from build123d import *

# Parameters (mm, degrees)
BOX010_W                = 100
BOX010_H                = 100
BOX010_DEPTH            = 20
CYLINDER010_R           = 6
CYLINDER010_DEPTH       = 60
CYLINDER011_R           = 2.1
CYLINDER011_DEPTH       = 40
BOX009_W                = 40
BOX009_H                = 30
BOX009_DEPTH            = 5
FILLET002_R             = 10
CYLINDER013_R           = 1
CYLINDER013_DEPTH       = 60
CYLINDER014_R           = 1
CYLINDER014_DEPTH       = 40
BODY005_PLACEMENT_ANGLE = 90
CYLINDER015_R           = 1
CYLINDER015_DEPTH       = 60
CYLINDER016_R           = 1
CYLINDER016_DEPTH       = 40
BODY006_PLACEMENT_ANGLE = 90
BOX008_W                = 22
BOX008_H                = 22
BOX008_DEPTH            = 50
CUT003_PLACEMENT_ANGLE  = 15


with BuildPart() as base_cube002:
    # Box010 → Box010 (new body)
    with BuildSketch(Plane(origin=(-8, -50, -20), x_dir=(1, 0, 0), z_dir=(0, 0, 1))):
        with Locations((50, 50)):
            Rectangle(BOX010_W, BOX010_H)
    extrude(amount=BOX010_DEPTH)


with BuildPart() as cone005:
    # Cone005 → Cone005 (revolve)
    with BuildSketch(Plane.XZ):
        Polygon((0, 0), (2.1, 0), (6, 4), (0, 4), align=None)
    revolve(axis=Axis((0, 0, 0), (0, 0, 1)))


with BuildPart() as cylinder010:
    # Cylinder010 → Cylinder010 (new body)
    with BuildSketch(Plane.XY.offset(4)):
        Circle(CYLINDER010_R)
    extrude(amount=CYLINDER010_DEPTH)


with BuildPart() as extraction_fusion001:
    # Cylinder011 → Cylinder011 (new body)
    with BuildSketch(Plane.XY.offset(-40)):
        Circle(CYLINDER011_R)
    extrude(amount=CYLINDER011_DEPTH)

    # Fusion012: union Cone005, Cylinder010
    add(cone005.part)
    add(cylinder010.part)


with BuildPart() as extraction_fusion001_1:
    # Fusion012 placement: moved
    add(extraction_fusion001.part.moved(Location((0, 0, 5))))


with BuildPart() as extraction_fusion001_2:
    # Body008 placement: moved
    add(extraction_fusion001_1.part.moved(Location((-17, 0, -5))))

    # Fusion014: union base cube002
    add(base_cube002.part)


with BuildPart() as base_cube_fillet001:
    # Box009 → Box009 (new body)
    with BuildSketch(Plane(origin=(-25, -15, 0), x_dir=(1, 0, 0), z_dir=(0, 0, 1))):
        with Locations((20, 15)):
            Rectangle(BOX009_W, BOX009_H)
    extrude(amount=BOX009_DEPTH)

    # Fillet002
    fillet002_edges = [base_cube_fillet001.edges().sort_by_distance(p)[0] for p in [
        (-25, -15, 2.5),
        (-25, 15, 2.5),
        (15, -15, 2.5),
        (15, 15, 2.5),
    ]]
    fillet(fillet002_edges, radius=FILLET002_R)


with BuildPart() as screw_hole_cylinder001:
    # Cylinder013 → Cylinder013 (new body)
    with BuildSketch(Plane.XY):
        Circle(CYLINDER013_R)
    extrude(amount=CYLINDER013_DEPTH)


with BuildPart() as m3_screw_hole_fusion_clone002:
    # Cylinder014 → Cylinder014 (new body)
    with BuildSketch(Plane.XY.offset(-40)):
        Circle(CYLINDER014_R)
    extrude(amount=CYLINDER014_DEPTH)

    # Fusion011: union screw hole cylinder001
    add(screw_hole_cylinder001.part)


with BuildPart() as m3_screw_hole_fusion_clone002_1:
    # Fusion011 placement: moved
    add(m3_screw_hole_fusion_clone002.part.moved(Location((0, 0, 5))))


with BuildPart() as m3_screw_hole_fusion_clone002_2:
    # Body005 placement: moved
    add(m3_screw_hole_fusion_clone002_1.part.moved(Location((11, 26, 37))).rotate(Axis((11, 26, 37), (1, 0, 0)), BODY005_PLACEMENT_ANGLE))


with BuildPart() as cylinder015:
    # Cylinder015 → Cylinder015 (new body)
    with BuildSketch(Plane.XY):
        Circle(CYLINDER015_R)
    extrude(amount=CYLINDER015_DEPTH)


with BuildPart() as m3_hole_fusion001:
    # Cylinder016 → Cylinder016 (new body)
    with BuildSketch(Plane.XY.offset(-40)):
        Circle(CYLINDER016_R)
    extrude(amount=CYLINDER016_DEPTH)

    # Fusion016: union Cylinder015
    add(cylinder015.part)


with BuildPart() as m3_hole_fusion001_1:
    # Fusion016 placement: moved
    add(m3_hole_fusion001.part.moved(Location((0, 0, 5))))


with BuildPart() as m3_hole_fusion001_2:
    # Body009 placement: moved
    add(m3_hole_fusion001_1.part.moved(Location((0, 0, -5))))


with BuildPart() as m3_hole_fusion001_3:
    # Clone006 placement: moved
    add(m3_hole_fusion001_2.part.moved(Location((0, 0, 10))))


with BuildPart() as m3_hole_fusion001_4:
    # Body006 placement: moved
    add(m3_hole_fusion001_3.part.moved(Location((-2, 11, 22))).rotate(Axis((-2, 11, 22), (0, 1, 0)), BODY006_PLACEMENT_ANGLE))

    # Fusion015: union m3 screw hole fusion clone002
    add(m3_screw_hole_fusion_clone002_2.part)


with BuildPart() as m3_hole_fusion001_5:
    # Fusion015 placement: moved
    add(m3_hole_fusion001_4.part.moved(Location((-7, 0, 0))))


with BuildPart() as stand_cut_v3:
    # Box008 → Box008 (new body)
    with BuildSketch(Plane(origin=(-7, 0, 0), x_dir=(1, 0, 0), z_dir=(0, 0, 1))):
        with Locations((11, 11)):
            Rectangle(BOX008_W, BOX008_H)
    extrude(amount=BOX008_DEPTH)

    # Cut003: cut m3 hole fusion001
    add(m3_hole_fusion001_5.part, mode=Mode.SUBTRACT)


with BuildPart() as stand_cut_v3_1:
    # Cut003 placement: moved
    add(stand_cut_v3.part.moved(Location((-2.27139, -11, 1.53433))).rotate(Axis((-2.27139, -11, 1.53433), (0, 1, 0)), CUT003_PLACEMENT_ANGLE))

    # Fusion013: union base cube fillet001
    add(base_cube_fillet001.part)

    # Cut004: cut extraction fusion001
    add(extraction_fusion001_2.part, mode=Mode.SUBTRACT)


solid = stand_cut_v3_1.part
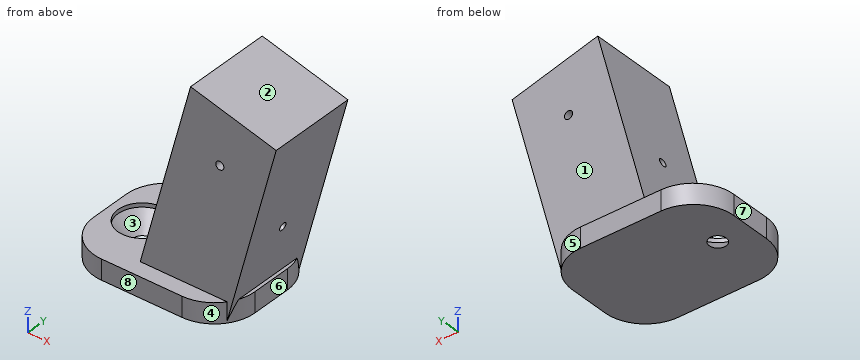
Geometry check sheet. Reference: the model listing, model coordinates, mm. Face numbers are marked on the shaded views. A direction names the side the tool comes from. Give positions to 0.01 mm unless a question says otherwise; leave off trailing zeros. Order: outer loops, then holes, each group sorted by start corner. A loop starts at its lowest first (then second) coordinate and runs counter-clockwise, first axis right, second up. Notation, with made-up numbers: (84.25, 23) - (102.25, 23) arc R23 ccw to (102.25, 41) - close; hole circle Ø6 at (27, 35.25). An arc over 180 degrees is marked (long way). Answer as a JSON object with one key per item and string values.
(1) Material ranges on line 1 (X direction, y = 0, z = 4.75); line 2 (Z direction, x = -12.5, y = 5); line 3 (Y direction, x = -2.5, z = 8), recorded low to high.
Report:
{"line 1": "-25 to -23, -11 to 15", "line 2": "0 to 5", "line 3": "-11 to 11"}
(2) Depth check by flat-ended pin: pin 1 Ø12 at (y, z) = (6, 33.5) entering from +X; pin 2 Ø1 at (y, z) = (9.5, 9.5) entering from +X; pin 3 Ø2 at (x, y) = (-14.5, 7) entering from +Z. Enter the tip coordinate at first touch or a pass-through.
Report:
{"pin 1": "x = 23.43", "pin 2": "x = 15.53", "pin 3": "z = 5"}
(3) Cross-section at A-A (y = 0). Record the cut outline in (x, z), then the cut area to 3 significant figures.
Report:
{"outline": "(-25, 0) - (-19.1, 0) - (-23, 4) - (-23, 5) - (-25, 5) - close; (-14.9, 0) - (15, 0) - (15, 5) - (14.19, 5) - (17.65, 17.94) - (-3.6, 23.63) - (-8.59, 5) - (-11, 5) - (-11, 4) - close; (-3.08, 25.56) - (18.17, 19.87) - (25.16, 45.95) - (3.91, 51.64) - close; hole circle Ø2 at (11.17, 36.24)", "area": "1,110 mm^2"}
(4) Cross-section at B-B (x = -17). Record the cut outline in (y, z), then the cut area to 3 significant figures.
Report:
{"outline": "(-14.8, 0) - (-2.1, 0) - (-6, 4) - (-6, 5) - (-14.8, 5) - close; (2.1, 0) - (14.8, 0) - (14.8, 5) - (6, 5) - (6, 4) - close", "area": "104 mm^2"}
(5) Tool access check on the marked faces 4, 5, 6, 7 and 8. Record the directions out of +Z, -Z, +X, -X, +Y, -Y that give a thin tool (end or side, any length) a straight path to the whole face; none if there is none.
Report:
{"face 4": "-Z, +X, -Y", "face 5": "-Z, +X, +Y", "face 6": "-Z, +X, +Y, -Y", "face 7": "+Z, -Z, -X, +Y, -Y", "face 8": "+Z, -Z, +X, -X, -Y"}
(6) Cross-section at C-C (x = -5). Record the cut outline in (y, z).
Report:
{"outline": "(-15, 0) - (15, 0) - (15, 5) - (11, 5) - (11, 18.4) - (-11, 18.4) - (-11, 5) - (-15, 5) - close"}
(7) Cross-section at D-D (y = 8). Record the cut outline in (x, z), then the cut area to 3 significant figures.
Report:
{"outline": "(-24.54, 0) - (14.54, 0) - (14.54, 5) - (14.19, 5) - (25.16, 45.95) - (3.91, 51.64) - (-8.59, 5) - (-24.54, 5) - close; hole circle Ø2 at (11.17, 36.24)", "area": "1,190 mm^2"}
(8) Draft check along X on the marked faces 1, 2 and 3. Enter one of: released by +X, released by -X, zero draft, split by the parting line, or undercut.
Report:
{"face 1": "zero draft", "face 2": "released by +X", "face 3": "undercut"}
